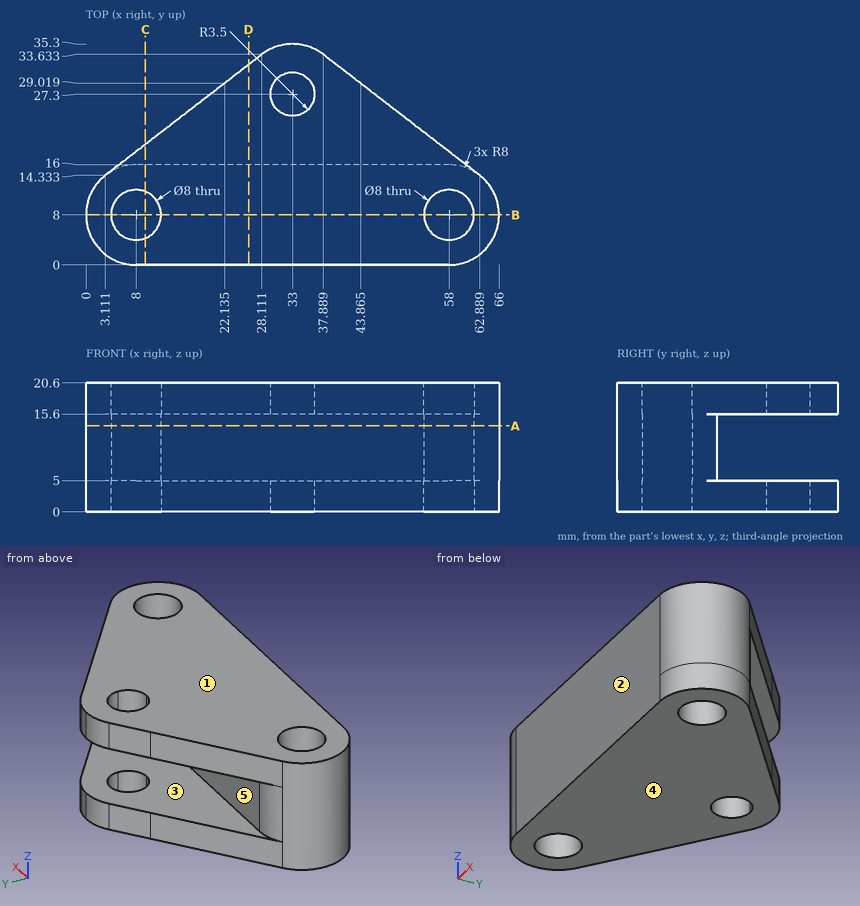
Design review of the part shown in the three views and the two pictorial views. Dimensions are in mm from the part's minimum x, y and z. A direction names the side the tool comes from. Give positions to 0.01 mm unless a question says otherwise; leave off trailing zeros. Loops run counter-clockwise (first coordinate to the right, second up) from the corner with the lowest first, then second, coordinate; pieces in that order, holes last. Notation, with made-up numbers: (-34.5, 21) -> (-1.5, 21) arc R17 cw to (-1.5, 40) -> close; hole circle Ø3 at (-39, 10). An arc over 180 degrees is marked (long way). Write each question's results on one line, items separated by ' | '.
1) Take a section at B-B, the plane y = 8. Give the boundary of the cut face in (x, z), plus the area to 3 significant figures.
Conclusion:
outline: (0, 0) -> (4, 0) -> (4, 20.6) -> (0, 20.6) -> close; (12, 0) -> (54, 0) -> (54, 20.6) -> (12, 20.6) -> close; (62, 0) -> (66, 0) -> (66, 20.6) -> (62, 20.6) -> close | area: 1,030 mm^2
2) For line 1 along X through (y, z) = (9, 9.25); line 2 along Z through (x, y) = (47.5, 25.5); line 3 along X through (y, z) = (6.5, 12.5), list the stretches that pass through material, from the lowest coordinate up. Write a range as from..to.
Conclusion:
line 1: x = 0.06..4.13, 11.87..54.13, 61.87..65.94 | line 2: z = 0..5, 15.6..20.6 | line 3: x = 0.14..4.29, 11.71..54.29, 61.71..65.86
3) Tool access review of the marked faces 4 and 5: name each direction out of +Z, -Z, +X, -X, +Y, -Y from which nothing blocks a thin tool from reaching the whole face with its end or side.
Conclusion:
face 4: -Z, +X, -X, +Y, -Y | face 5: +X, -X, +Y
4) Insertion check: pin 1 Ø3 at (x, z) = (13.5, 10) entering from +Y; pin 2 Ø7 at (x, y) = (8, 8) entering from -Z; pin 3 Ø6 at (y, z) = (13, 6) entering from +X; pin 4 Ø8.5 at (x, z) = (27, 12) entering from +Y. Each pin has a flat end and moves straight along its axis. Give the tip position at first contact, or say it passes through.
Conclusion:
pin 1: stops at y = 16 | pin 2: passes through | pin 3: stops at x = 65.75 | pin 4: stops at y = 34.37
5) Take a section at C-C, the plane x = 9.5. Give the boundary of the cut face in (y, z) (1 decimal).
Conclusion:
outline: (0, 0) -> (4.3, 0) -> (4.3, 20.6) -> (0, 20.6) -> close; (11.7, 0) -> (19.3, 0) -> (19.3, 5) -> (16, 5) -> (16, 15.6) -> (19.3, 15.6) -> (19.3, 20.6) -> (11.7, 20.6) -> close
6) Take a section at A-A, the plane z = 13.75. Give the boundary of the cut face in (x, y).
Conclusion:
outline: (8, 0) -> (58, 0) arc R8 ccw to (58, 16) -> (8, 16) arc R8 ccw to start; hole circle Ø8 at (8, 8); hole circle Ø8 at (58, 8)
7) Draft analysis for pull direction Z (two halves, no side actions). For the marked faces 1, 2 and 3, state which applies: pulls with the +Z half, pulls with the -Z half, needs draft (parallel to the pull), parting line crosses it, or undercut.
Conclusion:
face 1: pulls with the +Z half | face 2: needs draft | face 3: undercut
8) Take a section at D-D, the plane x = 26. Give the boundary of the cut face in (y, z).
Conclusion:
outline: (0, 0) -> (32, 0) -> (32, 5) -> (16, 5) -> (16, 15.6) -> (32, 15.6) -> (32, 20.6) -> (0, 20.6) -> close
